For this review, take the finished solid that the model builds, in its own axes (mm). Face numbers are marked on the shaded views. A direction names the side the tool comes from. Give positions to 0.01 mm unless a question says otherwise; leave off trailing zeros. Loops run counter-clockwise (first coordinate to the right, second up) from the corner with the lowest first, then second, coordinate; pieces in that order, holes last. Notation, with made-up numbers: (-7.5, 25.25) -> (26.5, 25.25) arc R23 ccw to (26.5, 45.25) -> close; hole circle Ø5 at (41, 55.5). An arc over 180 degrees is marked (long way). One line per question, with ' | ' between items. Start each with the question number.
(1) Consider section D-D (z = 2.75). Write out the cut boundary in (x, y), and give its area (3 significant figures).
(2) Tool access review of the marked faces 5, 6 and 7: name each direction out of +Z, -Z, +X, -X, +Y, -Y from which nothing blocks a thin tool from reaching the whole face with its end or side.
(3) Draft analysis for pull direction X (two halves, no side actions). For the marked faces 1, 2, 3 and 4, state which applies: +X half, -X half, draft (parallel to the pull), parting line (faces both ways), or undercut.
(4) Wall thickness on probe 1 along X at (y, z) = (10, 1.5); probe 2 along X at (y, z) = (43, 8.75); probe 3 along Y at (x, z) = (79.5, 14): over which ranges is each line inside the solid? List them lowest first.
(5) Consider section B-B (y = 42.85). Give the number of separate pieces and of enclosed holes in the cut face, and give its area (3 significant figures).
(6) Insertion check: P1, Ø13, axis at x = 17, y = 11, coming from the -Z side; P2, Ø5, axis at x = 14.5, y = 46, coming from the -Z side; P3, Ø11, axis at x = 20, y = 10, coming from the -Z side; P4, Ø5, axis at x = 81.5, y = 42.5, coming from the -Z side. Each pin has a flat end and moves straight along its axis. Give the tip position at first contact, or say it passes through.
(7) Consider section A-A (z = 10.75). Write out the cut boundary in (x, y).
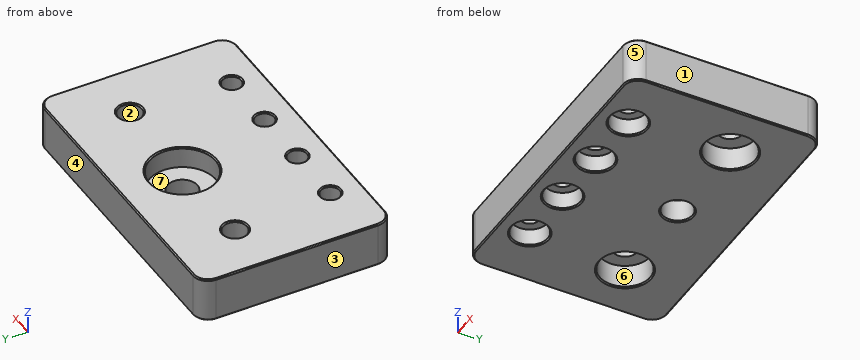
from build123d import *

# Parameters (mm, degrees)
SKETCH_W        = 100
SKETCH_H        = 64
SKETCH_R        = 5
SKETCH_R_2      = 3.2
SKETCH_R_3      = 4
PAD_DEPTH       = 15
SKETCH001_R     = 11.02
POCKET_DEPTH    = 7.2
SKETCH002_R     = 6
POCKET001_DEPTH = 6
SKETCH003_R     = 3.2
POCKET002_DEPTH = 15
SKETCH004_R     = 8.4
POCKET003_DEPTH = 8
FILLET_R        = 5
CHAMFER_SIZE    = 0.4
CHAMFER001_SIZE = 0.4


with BuildPart() as part:
    # Sketch → Pad (new body)
    with BuildSketch(Plane.XY):
        with Locations((50, 32)):
            Rectangle(SKETCH_W, SKETCH_H)
        with Locations((50, 42.85)):
            Circle(SKETCH_R, mode=Mode.SUBTRACT)
        with Locations((20, 10)):
            Circle(SKETCH_R_2, mode=Mode.SUBTRACT)
        with Locations((80, 10)):
            Circle(SKETCH_R_2, mode=Mode.SUBTRACT)
        with Locations((82, 42.85)):
            Circle(SKETCH_R_3, mode=Mode.SUBTRACT)
        with Locations((18, 42.85)):
            Circle(SKETCH_R_3, mode=Mode.SUBTRACT)
    extrude(amount=PAD_DEPTH)

    # Sketch001 (on Face11 of Pad) → Pocket (cut)
    with BuildSketch(Plane.XY.offset(15)):
        with Locations((50, 42.85)):
            Circle(SKETCH001_R)
    extrude(amount=-POCKET_DEPTH, mode=Mode.SUBTRACT)

    # Sketch002 (on Face4 of Pocket) → Pocket001 (cut)
    with BuildSketch(Plane(origin=(0, 0, 0), x_dir=(1, 0, 0), z_dir=(0, 0, -1))):
        with Locations((20, -10)):
            Circle(SKETCH002_R)
        with Locations((80, -10)):
            Circle(SKETCH002_R)
        with Locations((40, -10)):
            Circle(SKETCH002_R)
        with Locations((60, -10)):
            Circle(SKETCH002_R)
    extrude(amount=-POCKET001_DEPTH, mode=Mode.SUBTRACT)

    # Sketch003 (on Face5 of Pocket001) → Pocket002 (cut)
    with BuildSketch(Plane.XY.offset(15)):
        with Locations((40, 10)):
            Circle(SKETCH003_R)
        with Locations((60, 10)):
            Circle(SKETCH003_R)
    extrude(amount=-POCKET002_DEPTH, mode=Mode.SUBTRACT)

    # Sketch004 (on Face4 of Pocket002) → Pocket003 (cut)
    with BuildSketch(Plane(origin=(0, 0, 0), x_dir=(1, 0, 0), z_dir=(0, 0, -1))):
        with Locations((18, -42.85)):
            Circle(SKETCH004_R)
        with Locations((82, -42.85)):
            Circle(SKETCH004_R)
    extrude(amount=-POCKET003_DEPTH, mode=Mode.SUBTRACT)

    # Fillet
    fillet_edges = [part.edges().sort_by_distance(p)[0] for p in [
        (100, 0, 7.5),
        (0, 0, 7.5),
        (100, 64, 7.5),
        (0, 64, 7.5),
    ]]
    fillet(fillet_edges, radius=FILLET_R)

    # Chamfer
    chamfer_edges = [part.edges().sort_by_distance(p)[0] for p in [
        (50, 64, 15),
        (1.464466, 62.535534, 15),
        (98.535534, 62.535534, 15),
        (0, 32, 15),
        (100, 32, 15),
        (1.464466, 1.464466, 15),
        (98.535534, 1.464466, 15),
        (50, 0, 15),
        (76.8, 10, 15),
        (56.8, 10, 15),
        (36.8, 10, 15),
        (16.8, 10, 15),
        (78, 42.85, 15),
        (38.98, 42.85, 15),
        (14, 42.85, 15),
    ]]
    chamfer(chamfer_edges, length=CHAMFER_SIZE)

    # Chamfer001
    chamfer001_edges = [part.edges().sort_by_distance(p)[0] for p in [
        (50, 64, 0),
        (1.464466, 62.535534, 0),
        (98.535534, 62.535534, 0),
        (0, 32, 0),
        (100, 32, 0),
        (1.464466, 1.464466, 0),
        (98.535534, 1.464466, 0),
        (50, 0, 0),
        (74, 10, 0),
        (54, 10, 0),
        (34, 10, 0),
        (14, 10, 0),
        (73.6, 42.85, 0),
        (45, 42.85, 0),
        (9.6, 42.85, 0),
    ]]
    chamfer(chamfer001_edges, length=CHAMFER001_SIZE)


solid = part.part
A:
1) outline: (0, 5) arc R5 ccw to (5, 0) -> (95, 0) arc R5 ccw to (100, 5) -> (100, 59) arc R5 ccw to (95, 64) -> (5, 64) arc R5 ccw to (0, 59) -> close; hole circle Ø16.8 at (18, 42.85); hole circle Ø12 at (20, 10); hole circle Ø12 at (40, 10); hole circle Ø10 at (50, 42.85); hole circle Ø12 at (60, 10); hole circle Ø16.8 at (82, 42.85); hole circle Ø12 at (80, 10) | area: 5,400 mm^2
2) face 5: +Z, -Z, +X, -Y | face 6: -Z | face 7: +Z
3) face 1: +X half | face 2: undercut | face 3: -X half | face 4: draft
4) probe 1: x = 0 to 14, 26 to 34, 46 to 54, 66 to 74, 86 to 100 | probe 2: x = 0 to 14, 22 to 38.98, 61.02 to 78, 86 to 100 | probe 3: y = 0 to 6.84, 13.16 to 39.73, 45.97 to 64
5) separate pieces: 4 | enclosed holes: 0 | area: 881 mm^2
6) P1: stops at z = 0 | P2: stops at z = 8 | P3: stops at z = 6 | P4: passes through
7) outline: (0, 5) arc R5 ccw to (5, 0) -> (95, 0) arc R5 ccw to (100, 5) -> (100, 59) arc R5 ccw to (95, 64) -> (5, 64) arc R5 ccw to (0, 59) -> close; hole circle Ø8 at (18, 42.85); hole circle Ø6.4 at (20, 10); hole circle Ø6.4 at (40, 10); hole circle Ø22.04 at (50, 42.85); hole circle Ø6.4 at (60, 10); hole circle Ø6.4 at (80, 10); hole circle Ø8 at (82, 42.85)
